Here's how the part is built. I have some questions about the finished solid (model axes, mm). A direction names the side the tool comes from. Coordinates: 2 decimals unless noted, no trailing zeros. Write each loop counter-clockwise with the first axis right and the second up, starting at its lowest first coordinate (ties: lowest second). Pieces come first, ordered by that corner, then holes.
(1) Thinking about a two-plate mould opening in X: for faces 1 (the cylindrical face through (-48, 29, 2)), 2 (the flat face through (50, -29, -18)), 3 (the flat face through (-1, -30, -35)), 4 (the cylindrical face through (-36.23, -28.52, -45.93)), which applies, released by +X, released by -X, zero draft, split by the parting line, or undercut?
(2) Imagine slicing it at C-C, the plane z = -48.5. List the corners of the cut face in (x, y) for me, plus the area to 3 significant figures.
(3) Imagine slicing it at A-A, the plane x = -37.5. List the corners of the cut face in (y, z) for me.
(4) Imagine slicing it at B-B, the plane y = 10. List the corners of the cut face in (x, z) for me.
(5) Please list where these lines run through material, in increasing order: probe 1 along X at (y, z) = (10, 1); probe 2 along Z at (x, y) = (-19, 10); probe 3 along Y at (x, z) = (21.5, -42).
(6) Which directions (+Z, -Z, +X, -X, +Y, -Y) give clear straight access to the entire face, cutting with the end or side of a thin tool? Please do faces 5 (the flat face through (1, 30, 1)), 6 (the flat face through (-1, 5, 0)).
(7) Imagine slicing it at D-D, the plane x = 31.5. List the corners of the cut face in (y, z) for me, plus the area to 3 significant figures.
(8) For pin 1 Ø5.5 at (x, z) = (-37.5, -49) entering from +Y; pin 2 Ø8 at (x, z) = (-14, -48) entering from +Y; pin 3 Ø1 at (x, y) = (20.5, 3) entering from -Z, each with a flat end and sliding along its axis, tell me the tip position at first contact or that it passes through.
Autodesk Inventor part; units mm, degrees
ref_plane "YZ Plane" through (0, 0, 0) normal (1, 0, 0) x (0, 1, 0)
ref_plane "XZ Plane" through (0, 0, 0) normal (0, 1, 0) x (-1, 0, 0)
ref_plane "XY Plane" through (0, 0, 0) normal (0, 0, 1) x (1, 0, 0)
sketch "Sketch1" plane through (0, 0, 0) normal (0, 0, 1) x (1, 0, 0)
  line L0 (-50, -30) -> (50, -30)
  line L1 (50, -30) -> (50, 30)
  line L2 (50, 30) -> (-50, 30)
  line L3 (-50, 30) -> (-50, -30)
  line L4 (-50, -30) -> (50, 30) construction
  line L5 (50, -30) -> (-50, 30) construction
  point P0 (0, 0)
  dimension "d0" = 60
  dimension "d1" = 100
extrude "Extrusion1" add sketch "Sketch1" along normal blind 3
sketch "Sketch2" plane through (-50, -27, 3) normal (0, -1, 0) x (1, 0, 0)
  line L0 (100, 0) -> (0, 0)
  line L1 (0, 0) -> (0, -65)
  line L2 (0, -65) -> (100, -65)
  line L3 (100, -65) -> (100, 0)
edge flange "Flange1" height 65 angle 90 thickness 3 bend radius 7 thickness toward (0, -1, 0) relief tear relief width 3 relief depth 1.5 edges at (0, -30, 0) wall of the first edge with corners at (50, -27, 3) (-50, -27, 3) (-50, -27, -62) (50, -27, -62)
bend "Bend1"
corner "Corner1"
sketch "Sketch3" plane through (0, 0, 3) normal (0, 0, 1) x (1, 0, 0)
  line L0 (50, 30) -> (-50, 30)
  point P0 (0, 0)
  point P1 (-37.5, 10)
  point P2 (37.5, 10)
  dimension "d15" = 20
  dimension "d16" = 37.5
  dimension "d17" = 75
hole "Hole1" at (-37.5, 10, 3) at (37.5, 10, 3) direction (0, 0, -1) diameter 6.647 end through all
sketch "Sketch4" plane through (-50, -27, -62) normal (0, 1, 0) x (1, 0, 0)
  line L0 (0, -65) -> (100, -65)
  line L1 (50, -65) -> (50, 0) construction
  line L2 (100, 0) -> (0, 0)
  point P0 (50, -62)
  point P1 (87.5, -13)
  point P2 (12.5, -13)
  dimension "d26" = 37.5
  dimension "d27" = 75
  dimension "d36" = 52
hole "Hole2" at (37.5, -27, -49) at (-37.5, -27, -49) direction (0, -1, 0) diameter 6.647 end through all
fillet "Fillet1" radius 5 4 edges at (-50, 30, 1.5) (50, 30, 1.5) (-50, -28.5, -62) (50, -28.5, -62)
equation "\"d1\" = Width"
equation "\"d4\" = Thickness"
equation "\"d5\" = BendReliefWidth"
equation "\"d6\" = BendReliefDepth"
equation "\"d7\" = MinimumRemnant"
equation "\"d8\" = TransitionRadius"
equation "\"d12\" = CornerReliefSize"
equation "\"d13\" = GapSize"
equation "\"d14\" = JacobiRadiusSize"
equation "\"BendRadius\" = Thickness"
equation "\"BendReliefWidth\" = Thickness"
equation "\"BendReliefDepth\" = 0.5 * Thickness"
equation "\"CornerReliefSize\" = 4 * Thickness"
equation "\"MinimumRemnant\" = 2 * Thickness"
equation "\"TransitionRadius\" = BendRadius"
equation "\"JacobiRadiusSize\" = BendRadius"
equation "\"GapSize\" = Thickness"
properties part number "Clamp_Plate" material "Steel, Carbon"
Recorded:
1. face 1: released by -X
1. face 2: released by +X
1. face 3: zero draft
1. face 4: undercut
2. outline: (-50, -30) - (-40.79, -30) - (-40.79, -27) - (-50, -27) - close; (-34.21, -30) - (34.21, -30) - (34.21, -27) - (-34.21, -27) - close; (40.79, -30) - (50, -30) - (50, -27) - (40.79, -27) - close
2. area: 261 mm2
3. outline: (-30, -62) - (-27, -62) - (-27, -52.32) - (-30, -52.32) - close; (-30, -45.68) - (-27, -45.68) - (-27, -7) arc R7 cw to (-20, 0) - (6.68, 0) - (6.68, 3) - (-20, 3) arc R10 ccw to (-30, -7) - close; (13.32, 0) - (30, 0) - (30, 3) - (13.32, 3) - close
4. outline: (-50, 0) - (-40.82, 0) - (-40.82, 3) - (-50, 3) - close; (-34.18, 0) - (34.18, 0) - (34.18, 3) - (-34.18, 3) - close; (40.82, 0) - (50, 0) - (50, 3) - (40.82, 3) - close
5. probe 1: x = -50 to -40.82, -34.18 to 34.18, 40.82 to 50
5. probe 2: z = 0 to 3
5. probe 3: y = -30 to -27
6. face 5: +Z, -Z, +X, -X, +Y
6. face 6: -Z, +X, -X, +Y
7. outline: (-30, -62) - (-27, -62) - (-27, -7) arc R7 cw to (-20, 0) - (30, 0) - (30, 3) - (-20, 3) arc R10 ccw to (-30, -7) - close
7. area: 355 mm2
8. pin 1: passes through
8. pin 2: stops at y = -27
8. pin 3: stops at z = 0
